The model under review builds one solid part; all positions refer to its coordinate system, in mm. A direction names the side the tool comes from. Round coordinates to 2 decimals unless told otherwise and drop trailing zeros. Order: outer loops, then holes, each group sorted by start corner. A loop starts at its lowest first (then second) coordinate and runs counter-clockwise, first axis right, second up. Notation, with made-up numbers: M 28.25,80.25 L 40.25,80.25 A15 cw 40.25,106.25 Z; hole C 46,16 d8. An arc over 180 degrees is marked long. One line per item, written item: value. Start each with the question number.
from build123d import *

# Parameters (mm, degrees)
F1_DEPTH = 5
F2_R     = 3
F3_DEPTH = 15
F4_R     = 2
F5_DEPTH = 1
F6_R     = 3
F6_R_2   = 2
F7_DEPTH = 7


with BuildPart() as f1:
    # F0 (on Top) → F1 (new body)
    with BuildSketch(Plane.XY):
        with BuildLine():
            ThreePointArc((0, -7.5), (5.3033008589, -5.3033008589), (7.5, 0))
            ThreePointArc((7.5, 0), (7.0062926922, 2.6761656733), (5.5901699437, 5))
            Line((5.5901699437, 5), (-5.5901699437, 5))
            ThreePointArc((-5.5901699437, 5), (-7.0062926922, 2.6761656733), (-7.5, 0))
            ThreePointArc((-7.5, 0), (-5.3033008589, -5.3033008589), (0, -7.5))
        make_face()
        with BuildLine():
            Line((7.5, -7.5), (7.5, 0))
            ThreePointArc((7.5, 0), (5.3033008589, -5.3033008589), (0, -7.5))
            Line((0, -7.5), (7.5, -7.5))
        make_face()
        with BuildLine():
            Line((-7.5, -7.5), (0, -7.5))
            ThreePointArc((0, -7.5), (-5.3033008589, -5.3033008589), (-7.5, 0))
            Line((-7.5, 0), (-7.5, -7.5))
        make_face()
        with BuildLine():
            Line((7.5, -7.5), (0, -7.5))
            ThreePointArc((0, -7.5), (3.5355339059, -8.9644660941), (5, -12.5))
            Line((5, -12.5), (7.5, -12.5))
            Line((7.5, -12.5), (7.5, -7.5))
        make_face()
        with BuildLine():
            ThreePointArc((-5, -12.5), (-3.5355339059, -8.9644660941), (0, -7.5))
            Line((0, -7.5), (-7.5, -7.5))
            Line((-7.5, -7.5), (-7.5, -12.5))
            Line((-7.5, -12.5), (-5, -12.5))
        make_face()
    extrude(amount=F1_DEPTH)

    # F2 (on face) → F3 (join)
    with BuildSketch(Plane(origin=(0, 0, 0), x_dir=(1, 0, 0), z_dir=(0, 0, -1))):
        Circle(F2_R)
    extrude(amount=F3_DEPTH)

    # F4 (on face) → F5 (join)
    with BuildSketch(Plane(origin=(0, 0, -15), x_dir=(1, 0, 0), z_dir=(0, 0, -1))):
        Circle(F4_R)
    extrude(amount=F5_DEPTH)

    # F6 (on face) → F7 (join)
    with BuildSketch(Plane(origin=(0, 0, -16), x_dir=(1, 0, 0), z_dir=(0, 0, -1))):
        Circle(F6_R)
        Circle(F6_R_2, mode=Mode.SUBTRACT)
        Circle(F6_R_2)
    extrude(amount=F7_DEPTH)


solid = f1.part
Item 1: The part is to be moulded in two halves that separate along Z. For faces 1 (the flat face through (7.5, -6, 2)), 2 (the flat face through (0, -4, 5)), 3 (the flat face through (1, 2, -16)), 4 (the flat face through (0, 0, -23)), say which applies: pulls with the +Z half, pulls with the -Z half, needs draft (parallel to the pull), parting line crosses it, or undercut.
Item 2: Consider section B-B, the plane x = 2.5. Give the boundary of the cut face in (y, z).
Item 3: Clearance check with flat-ended pins moving along their axes: P1, Ø5, axis at x = -3.5, y = -4, coming from the -Z side; P2, Ø10, axis at y = -2.5, z = -7, coming from the +X side; P3, Ø5, axis at x = -4.5, z = -7.5, coming from the -Y side; P4, Ø1.5, axis at x = -2.5, z = -7.5, coming from the -Y side. State where each tip first meets the part, or that it passes through.
Item 4: Consider section D-D, the plane y = -8.25. Give the boundary of the cut face in (x, z), then the cut area to 3 significant figures.
Item 5: Machinability: for faces 5 (the flat face through (6, -12.5, 2)), 6 (the cylindrical face through (-3, 0, -19)), 7 (the cylindrical face through (-0.434, 1.952, -15.493)), which of the approach directions +Z, -Z, +X, -X, +Y, -Y give a long, thin tool a straight path to every point of the face, cutting with its end or side? Answer none if there is none.
Item 6: Consider section A-A, the plane z = 1.25. Give the boundary of the cut face in (x, y).
Item 7: Consider section C-C, the plane y = -1.25. Give the boundary of the cut face in (x, z).
Item 8: Wall thickness on L1, parallel to Z at x = -4.5, y = 1.75; L2, parallel to Z at x = 2, y = -1.25; L3, parallel to X at y = -2, z = -13.5: over which ranges is each line inside the solid? List them lowest first.
Computed:
1. face 1: needs draft
1. face 2: pulls with the +Z half
1. face 3: undercut
1. face 4: pulls with the -Z half
2. outline: M -8.17,0 L -1.66,0 L -1.66,-15 L 1.66,-15 L 1.66,0 L 5,0 L 5,5 L -8.17,5 Z; M -1.66,-23 L 1.66,-23 L 1.66,-16 L -1.66,-16 Z
3. P1: stops at z = -23
3. P2: stops at x = 3
3. P3: stops at y = -2.24
3. P4: stops at y = -2.44
4. outline: M -7.5,0 L -2.63,0 L -2.63,5 L -7.5,5 Z; M 2.63,0 L 7.5,0 L 7.5,5 L 2.63,5 Z
4. area: 48.7 mm^2
5. face 5: +Z, -Z, +X, -X, -Y
5. face 6: -Z
5. face 7: none
6. outline: M -7.5,-12.5 L -5,-12.5 A5 cw 5,-12.5 L 7.5,-12.5 L 7.5,0 A7.5 ccw 5.59,5 L -5.59,5 A7.5 ccw -7.5,0 Z
7. outline: M -7.5,0 L -2.73,0 L -2.73,-15 L -1.56,-15 L -1.56,-16 L -2.73,-16 L -2.73,-23 L 2.73,-23 L 2.73,-16 L 1.56,-16 L 1.56,-15 L 2.73,-15 L 2.73,0 L 7.5,0 L 7.5,5 L -7.5,5 Z
8. L1: z = 0 to 5
8. L2: z = -23 to -16, -15 to 5
8. L3: x = -2.24 to 2.24
